from build123d import *


with BuildPart() as part:
    # Croquis1 → Revolución1 (revolve)
    with BuildSketch(Plane(origin=(0, 0, 0), x_dir=(1, 0, 0), z_dir=(0, 1, 0))):
        with BuildLine():
            Line((0, 6), (18, 6))
            ThreePointArc((18, 6), (22.102949779, 4.89077105), (25.088082902, 1.865284974))
            ThreePointArc((25.088082902, 1.865284974), (25.079723626, 0.620161218), (24, 0))
            Line((24, 0), (21, 0))
            Line((21, 0), (21, 1))
            Line((21, 1), (22, 1))
            Line((22, 1), (22, 4))
            Line((22, 4), (0, 4))
            Line((0, 4), (0, 6))
        make_face()
    revolve(axis=Axis((0, 0, 0), (0, 0, -1)))


solid = part.part
Input: part model. Units: mm. Frame: model coordinates. A direction names the side the tool comes from. Coordinates: 2 decimals unless noted, no trailing zeros. Order: outer loops, then holes, each group sorted by start corner. A loop starts at its lowest first (then second) coordinate and runs counter-clockwise, first axis right, second up.
1. Access query for faces 4 (the flat face through (0, 0, -6)), 5 (the cylindrical face through (-4.769, 21.477, -2.521)). Directions: +Z, -Z, +X, -X, +Y, -Y. A direction counts if a zero-diameter tool reaches every point of the face in a straight line with its end or side. Return the directions, or none.
Checked values:
face 4: -Z, +X, -X, +Y, -Y
face 5: none
2. Draft query along X for faces 1 (the flat face through (0, 0, -4)), 2 (the flat face through (-0.1, 21.2, 0)), 3 (the cylindrical face through (20.03, -6.31, -0.51)). Return one class per face: +X half, -X half, draft (parallel to the pull), parting line (faces both ways), or undercut.
Checked values:
face 1: undercut
face 2: draft
face 3: undercut
3. Contact query for flat-ended pins moving along their axis: P1, Ø1, axis at x = 11, y = 17.5, coming from the -Z side; P2, Ø13, axis at x = 2, y = 9.5, coming from the +Z side. Output: stop coordinate, or through.
Checked values:
P1: stops at z = -5.71
P2: stops at z = -4
4. Cut plane C-C, the plane z = -4.75. Return loops of the section in (x, y), plus the area to 3 significant figures.
Checked values:
outline: circle Ø44.67 at (0, 0)
area: 1,570 mm2
5. Ray query, line 1 along Y through (x, z) = (0, -0.65); line 2 along Z through (x, y) = (3, 6); line 3 along X through (y, z) = (-7, -2.5). Return the intervals inside material, ascending.
Checked values:
line 1: y = -25.1 to -21, 21 to 25.1
line 2: z = -6 to -4
line 3: x = -23.68 to -20.86, 20.86 to 23.68
6. Cut plane A-A, the plane y = 0. Return loops of the section in (x, z).
Checked values:
outline: (-25.09, -1.87) arc R8.14 ccw to (-18, -6) - (18, -6) arc R8.14 ccw to (25.09, -1.87) arc R1.25 ccw to (24, 0) - (21, 0) - (21, -1) - (22, -1) - (22, -4) - (-22, -4) - (-22, -1) - (-21, -1) - (-21, 0) - (-24, 0) arc R1.25 ccw to start
